Input: part model. Units: mm. Frame: model coordinates. Face numbers are marked on the shaded views. A direction names the side the tool comes from. Give positions to 0.01 mm unless a question says otherwise; leave off trailing zeros. Write each loop counter-clockwise with the first axis right and the second up, starting at its lowest first coordinate (ties: lowest second). Pieces come first, ordered by that corner, then holes. Notation, with made-up numbers: (-13.5, 89) - (2.5, 89) arc R14 cw to (2.5, 110) - close; hole circle Ø10 at (0.25, 3). An arc over 180 degrees is marked (long way). Use a Markdown table: item, result. Add a question column.
1. Section query A-A, the plane z = 10. Return loops of the section in (x, y).
2. Pin query (flat end, axial travel): pin 1 (6 mm diameter, centred on x = -68, z = 9.5, fed in from +Y); pin 2 (5 mm diameter, centred on y = 49.5, z = 15, fed in from +X); pin 3 (1.5 mm diameter, centred on y = 50, z = 2.5, fed in from -X). Return the tip coordinate at first contact, or that it passes through.
3. Section query B-B, the plane x = -65. Return loops of the section in (y, z).
4. Set-up query: the marked faces 1, 2 and 3. Return all of +Z, -Z, +X, -X, +Y, -Y with unobstructed straight access to the full face (end or side cutting, diameter ignored); none if empty.
5. Section query D-D, the plane y = 51.5. Return loops of the section in (x, z).
6. Material intervals for probe 1 along X at (y, z) = (8, 9.75); probe 2 along Z at (x, y) = (65, 11.5); probe 3 along Z at (x, y) = (65, 18), sorted ascending.
7. Section query C-C, the plane z = 2. Return loops of the section in (x, y), plus the area to 3 significant figures.
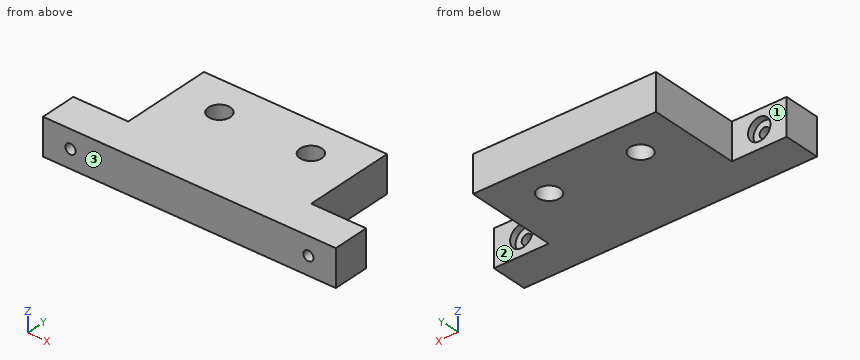
```python
from build123d import *

# Parameters (mm, degrees)
SKETCH2_R              = 6
CORPO_FUROS_12MM_DEPTH = 20
FUROS_6MM_D            = 5.5
FUROS_6MM_CBORE_D      = 12.24
FUROS_6MM_CBORE_DEPTH  = 3.58


with BuildPart() as part:
    # Sketch2 → Corpo - Furos 12mm (new body)
    with BuildSketch(Plane.XY):
        Polygon((80, 0), (-80, 0), (-80, 20), (-50, 20), (-50, 70), (0, 70), (50, 70), (50, 20), (80, 20), align=None)
        with Locations((-25, 50)):
            Circle(SKETCH2_R, mode=Mode.SUBTRACT)
        with Locations(Location((25, 50, 0), (0, 0, 180))):
            Circle(SKETCH2_R, mode=Mode.SUBTRACT)
    extrude(amount=CORPO_FUROS_12MM_DEPTH)

    # Furos Ø6mm (through all)
    with Locations(Plane(origin=(0, 20, 0), x_dir=(1, 0, 0), z_dir=(0, 1, 0))):
        with Locations((-65, -10), (65, -10)):
            CounterBoreHole(FUROS_6MM_D / 2, FUROS_6MM_CBORE_D / 2, FUROS_6MM_CBORE_DEPTH)


solid = part.part
```
Result sheet:
| question | item | result |
|---|---|---|
| 1 | outline | (-80, 0) - (-67.75, 0) - (-67.75, 16.42) - (-71.12, 16.42) - (-71.12, 20) - (-80, 20) - close; (-62.25, 0) - (62.25, 0) - (62.25, 16.42) - (58.88, 16.42) - (58.88, 20) - (50, 20) - (50, 70) - (-50, 70) - (-50, 20) - (-58.88, 20) - (-58.88, 16.42) - (-62.25, 16.42) - close; (67.75, 0) - (80, 0) - (80, 20) - (71.12, 20) - (71.12, 16.42) - (67.75, 16.42) - close; hole circle Ø12 at (-25, 50); hole circle Ø12 at (25, 50) |
| 2 | pin 1 | stops at y = 16.42 |
| 2 | pin 2 | stops at x = 50 |
| 2 | pin 3 | stops at x = -50 |
| 3 | outline | (0, 0) - (20, 0) - (20, 3.88) - (16.42, 3.88) - (16.42, 7.25) - (0, 7.25) - close; (0, 12.75) - (16.42, 12.75) - (16.42, 16.12) - (20, 16.12) - (20, 20) - (0, 20) - close |
| 4 | face 1 | +Z, -Z, -X, +Y |
| 4 | face 2 | +Z, -Z, +X, +Y |
| 4 | face 3 | +Z, -Z, +X, -X, -Y |
| 5 | outline | (-50, 0) - (-30.81, 0) - (-30.81, 20) - (-50, 20) - close; (-19.19, 0) - (19.19, 0) - (19.19, 20) - (-19.19, 20) - close; (30.81, 0) - (50, 0) - (50, 20) - (30.81, 20) - close |
| 6 | probe 1 | x = -80 to -67.74, -62.26 to 62.26, 67.74 to 80 |
| 6 | probe 2 | z = 0 to 7.25, 12.75 to 20 |
| 6 | probe 3 | z = 0 to 3.88, 16.12 to 20 |
| 7 | outline | (-80, 0) - (80, 0) - (80, 20) - (50, 20) - (50, 70) - (-50, 70) - (-50, 20) - (-80, 20) - close; hole circle Ø12 at (-25, 50); hole circle Ø12 at (25, 50) |
| 7 | area | 7,970 mm² |
